```python
from build123d import *

# Parameters (mm, degrees)
SKETCH2_R           = 1.6
BOSS_EXTRUDE1_DEPTH = 17
SKETCH2_17_R        = 1.6
BOSS_EXTRUDE2_DEPTH = 6
CUT_EXTRUDE1_DEPTH  = 3
CUT_EXTRUDE2_DEPTH  = 3
FILLET1_R           = 1.5
CHAMFER3_SIZE       = 1


# Some blends are built 0.0001 mm under size
with BuildPart() as part:
    # Sketch2 → Boss-Extrude1 (new body)
    with BuildSketch(Plane.XY):
        Polygon((-47.316130455, 164.5), (-52.0477435, 177.5), (-55.240276817, 177.5), (-119.71566449, 354.644671741), (-104.09954666, 354.644671741), (-104.09954666, 349.79492948), (-101.29954666, 348.178348727), (-98.49954666, 349.79492948), (-98.49954666, 354.644671741), (-86.075962148, 354.644671741), (-16.868961429, 164.5), (-13.676428112, 164.5), (-83.975339533, 357.644671741), (-124.00010851, 357.644671741), (-53.701197089, 164.5), align=None)
        with Locations((-101.29954666, 351.411510234)):
            Circle(SKETCH2_R, mode=Mode.SUBTRACT)
    extrude(amount=-BOSS_EXTRUDE1_DEPTH)

    # Sketch2<17> → Boss-Extrude2 (add)
    with BuildSketch(Plane.XY):
        Polygon((-52.0477435, 177.5), (-47.316130455, 164.5), (-16.868961429, 164.5), (-86.075962148, 354.644671741), (-98.49954666, 354.644671741), (-98.49954666, 349.79492948), (-101.29954666, 348.178348727), (-104.09954666, 349.79492948), (-104.09954666, 354.644671741), (-119.71566449, 354.644671741), (-55.240276817, 177.5), align=None)
        with Locations((-44.822322699, 172)):
            Circle(SKETCH2_17_R, mode=Mode.SUBTRACT)
        with Locations((-24.822322699, 172)):
            Circle(SKETCH2_17_R, mode=Mode.SUBTRACT)
    extrude(amount=-BOSS_EXTRUDE2_DEPTH)

    # Sketch2<18> → Cut-Extrude1 (cut)
    with BuildSketch(Plane.XY):
        Polygon((-24.822322699, 168.766838493), (-22.022322699, 170.383419246), (-22.022322699, 173.616580754), (-24.822322699, 175.233161507), (-27.622322699, 173.616580754), (-27.622322699, 170.383419246), align=None)
        Polygon((-44.822322699, 168.766838493), (-42.022322699, 170.383419246), (-42.022322699, 173.616580754), (-44.822322699, 175.233161507), (-47.622322699, 173.616580754), (-47.622322699, 170.383419246), align=None)
        Polygon((-101.29954666, 354.644671741), (-104.09954666, 353.028090988), (-104.09954666, 349.79492948), (-101.29954666, 348.178348727), (-98.49954666, 349.79492948), (-98.49954666, 353.028090988), align=None)
    extrude(amount=-CUT_EXTRUDE1_DEPTH, mode=Mode.SUBTRACT)

    # Sketch5 → Cut-Extrude2 (cut)
    with BuildSketch(Plane.XY):
        Polygon((-118.540554996, 342.644671741), (-78.515786019, 342.644671741), (-19.135981626, 179.5), (-59.160750603, 179.5), align=None)
    extrude(amount=-CUT_EXTRUDE2_DEPTH, mode=Mode.SUBTRACT)

    # Fillet1
    fillet1_edges = [part.edges().sort_by_distance(p)[0] for p in [
        (-121.270331753, 350.144671741, 0),
        (-81.245562776, 350.144671741, 0),
        (-39.148366115, 179.5, 0),
        (-98.528170508, 342.644671741, 0),
        (-98.528170508, 342.644671741, -3),
        (-39.148366115, 179.5, -3),
        (-56.430973846, 172, 0),
        (-103.987724022, 357.644671741, 0),
        (-16.406204869, 172, 0),
        (-33.688812601, 164.5, 0),
        (-53.701197089, 164.5, -8.5),
        (-124.00010851, 357.644671741, -8.5),
        (-83.975339533, 357.644671741, -8.5),
    ]]
    fillet(fillet1_edges, radius=FILLET1_R - 0.0001)  # a hair under: the kernel refuses the full size

    # Chamfer2
    # the kernel refuses this chamfer: 3.34631437, 2 mm, written as the material it adds along each edge
    with BuildSketch(Plane(origin=(-55.240276817, 177.5, -6), x_dir=(0.9998669641130704, -0.01631116413110759, 0), z_dir=(0, 0, -1))) as chamfer2_piece_1_section:
        with BuildLine():
            Line((3.468087381, 0), (-0.836822437, -1.922560005))
            Line((-0.836822437, -1.922560005), (-0.899330844, -1.898647101))
            ThreePointArc((-0.899330844, -1.898647101), (-0.436719507, -0.954276075), (-0.062508407, 0.023912905))
            Line((-0.062508407, 0.023912905), (0.001091646, 0.066917384))
            ThreePointArc((0.001091646, 0.066917384), (1.734673987, 0.038636875), (3.469179027, 0.066917384))
            Line((3.469179027, 0.066917384), (3.468087381, 0))
        make_face()
    chamfer2_piece_1 = extrude(amount=11, mode=Mode.PRIVATE)
    chamfer2_piece_1 = split(chamfer2_piece_1, bisect_by=Plane(origin=(-52.5138481, 178.780611864, -11.5), z_dir=(-0.9396926207859072, -0.34202014332567215, 0)), keep=Keep.TOP, mode=Mode.PRIVATE)
    add(chamfer2_piece_1)

    # Chamfer3
    chamfer3_edges = [part.edges().sort_by_distance(p)[0] for p in [
        (-87.819990797, 267.012028492, -17),
        (-111.907605575, 354.644671741, -17),
    ]]
    chamfer(chamfer3_edges, length=CHAMFER3_SIZE)


solid = part.part
```
The model under review builds one solid part; all positions refer to its coordinate system, in mm. A direction names the side the tool comes from. Give positions to 0.01 mm unless a question says otherwise; leave off trailing zeros. Loops run counter-clockwise (first coordinate to the right, second up) from the corner with the lowest first, then second, coordinate; pieces in that order, holes last. Notation, with made-up numbers: (15, 87) - (74, 87) arc R11 cw to (74, 108) - close; hole circle Ø10 at (53, 26.5). An arc over 180 degrees is marked (long way). Answer as a JSON object with one key per item and string values.
Q1. For faces 1 (the flat face through (-103, 350, -3)), 2 (the flat face through (-98.5, 352, -11)), 3 (the flat face through (-37, 172, 0)), list the 3-axis set-ups (+Z, -Z, +X, -X, +Y, -Y) from which the entire face can be reached by the end or side of a thin tool; tool diameter is ignored.
Worked out:
{"face 1": "+Z", "face 2": "-Z", "face 3": "+Z, +X, -X, +Y, -Y"}
Q2. Insertion check: pin 1 (3 mm diameter, centred on y = 353, z = -9, fed in from -X); pin 2 (2.5 mm diameter, centred on y = 352, z = -2, fed in from -X); pin 3 (4 mm diameter, centred on x = -101.3, y = 351.41, fed in from +Z). Each pin has a flat end and moves straight along its axis. Give the tip position at first contact, or say it passes through.
Worked out:
{"pin 1": "stops at x = -122.86", "pin 2": "stops at x = -122.4", "pin 3": "stops at z = -3"}
Q3. To check wall thickness, follow line 1 along X through (y, z) = (172, -4.2); line 2 along X through (y, z) = (259.5, -7.25); line 3 along X through (y, z) = (225, -9.5). State the ranges of each line that lie inside material, in increasing order.
Worked out:
{"line 1": "x = -56.43 to -46.42, -43.22 to -26.42, -23.22 to -16.41", "line 2": "x = -88.28 to -85.09, -51.45 to -48.25", "line 3": "x = -75.72 to -72.53, -38.89 to -35.7"}
Q4. Mouldability with a two-part tool opening along X and no side actions: class faces 4 (the flat face through (-68, 262, -3)), 5 (the flat face through (-46.1, 170.6, -3)), 6 (the flat face through (-69, 260, -6)), 7 (the cylindrical face through (-81.504, 349.603, -0.451)) as +X half, -X half, draft (parallel to the pull), parting line (faces both ways), or undercut.
Worked out:
{"face 4": "draft", "face 5": "undercut", "face 6": "undercut", "face 7": "+X half"}
Q5. Add section B-B on z = -13.5. State the section outline as (x, y) points.
Worked out:
{"outline": "(-123.27, 355.63) - (-54.06, 165.49) arc R1.5 ccw to (-52.65, 164.5) - (-47.32, 164.5) - (-52.08, 177.59) - (-55.92, 179.38) - (-119.72, 354.64) - (-104.1, 354.64) - (-104.1, 349.79) - (-101.3, 348.18) - (-98.5, 349.79) - (-98.5, 354.64) - (-86.08, 354.64) - (-16.87, 164.5) - (-13.68, 164.5) - (-83.62, 356.66) arc R1.5 ccw to (-85.03, 357.64) - (-121.86, 357.64) arc R1.5 ccw to start; hole circle Ø3.2 at (-101.3, 351.41)"}
Q6. Add section A-A on x = -61.5. State the section outline as (y, z) points, plus the area to 3 significant figures.
Worked out:
{"outline": "(185.93, -17) - (191.77, -17) - (194.7, -16) - (194.7, -6) - (287.12, -6) - (287.12, -17) - (295.89, -17) - (295.89, -3) - (185.93, -3) - close", "area": "521 mm^2"}
Q7. Add section C-C on y = 210.5. State the section outline as (x, z) points, plus the area to 3 significant figures.
Worked out:
{"outline": "(-70.44, -17) - (-68.32, -17) - (-67.25, -16) - (-67.25, -6) - (-33.61, -6) - (-33.61, -17) - (-30.42, -17) - (-30.42, -3) - (-70.44, -3) - close", "area": "190 mm^2"}
